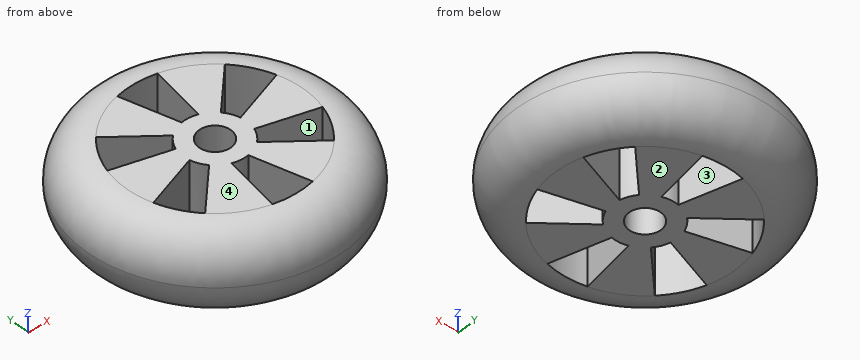
from build123d import *

# Parameters (mm, degrees)
SKETCH_1_R               = 32.5
SKETCH_1_R_2             = 4
EXTRUDE_1_DEPTH          = 20
FILLET_1_R               = 10
CUT_EXTRUDE_1_DEPTH      = 20
PATTERN_CIRCULAR_1_COUNT = 6


with BuildPart() as part:
    # 草图1 → 凸台-拉伸1 (new body)
    with BuildSketch(Plane.XY):
        Circle(SKETCH_1_R)
        Circle(SKETCH_1_R_2, mode=Mode.SUBTRACT)
    extrude(amount=EXTRUDE_1_DEPTH)

    # 圆角1
    fillet_1_edges = [part.edges().sort_by_distance(p)[0] for p in [
        (-32.5, 0, 0),
        (-32.5, 0, 20),
    ]]
    fillet(fillet_1_edges, radius=FILLET_1_R - 0.0001)  # a hair under: the kernel refuses the full size

    # 草图2 → 切除-拉伸1 (cut)
    with BuildSketch(Plane.XY.offset(20)):
        with BuildLine():
            Line((-5.142061575, 21.884386505), (-1.389185421, 7.878462024))
            ThreePointArc((-1.389185421, 7.878462024), (0.633872, 7.974848355), (2.616301677, 7.560090313))
            Line((2.616301677, 7.560090313), (5.142061575, 21.884386505))
            ThreePointArc((5.142061575, 21.884386505), (0, 22.480372994), (-5.142061575, 21.884386505))
        make_face()
    cut_extrude_1 = extrude(amount=-CUT_EXTRUDE_1_DEPTH, mode=Mode.SUBTRACT)

    # 阵列(圆周)1: 切除-拉伸1 ×6 about axis
    pattern_circular_1_axis = Axis((0, 0, 0), (0, 0, 1))
    for i in range(1, PATTERN_CIRCULAR_1_COUNT):
        add(cut_extrude_1.rotate(pattern_circular_1_axis, i * 360 / PATTERN_CIRCULAR_1_COUNT), mode=Mode.SUBTRACT)


solid = part.part
Build history of the part. All positions in model axes, mm. Face numbers are marked on the shaded views. A direction names the side the tool comes from. Round coordinates to 2 decimals unless told otherwise and drop trailing zeros. Loops run counter-clockwise (first coordinate to the right, second up) from the corner with the lowest first, then second, coordinate; pieces in that order, holes last. Notation, with made-up numbers: (22.25, 18.5) -> (65.25, 18.5) arc R25 ccw to (65.25, 38.5) -> close; hole circle Ø5 at (88.25, 13.5). An arc over 180 degrees is marked (long way). Answer in a Markdown table with one row per item.
Item 1: Saw through at B-B (x = 0). State how many separate pieces and enclosed holes the cut face has, and give its area (3 significant figures).
Answers below:
| item | result |
|---|---|
| separate pieces | 4 |
| enclosed holes | 0 |
| area | 475 mm² |
Item 2: Which spindle directions (+Z, -Z, +X, -X, +Y, -Y) get a long thin tool onto all of the face, cutting with end or side? Do the marked faces 3 and 4. Say none if no direction does.
Answers below:
| item | result |
|---|---|
| face 3 | +Z, -Z |
| face 4 | +Z, +X, -X, +Y, -Y |
Item 3: Drill centre lines: L1, parallel to Y at x = 10.5, z = 14; L2, parallel to Y at x = 1, z = 1.25; L3, parallel to Y at x = -15, z = 8.5. Where is each one in solid material? Low to high. Write a range as [from, to].
Answers below:
| item | result |
|---|---|
| L1 | y = [-29.87, -10.46], [-3.54, 2.48], [9.51, 29.87] |
| L2 | y = [-27.32, -22.46], [-7.94, -3.87], [3.87, 7.94], [22.46, 27.32] |
| L3 | y = [-28.7, -14.01], [-4.11, 4.74], [14.24, 28.7] |
Item 4: Pin check, flat tips, straight feed: pin 1 (9 mm diameter, centred on x = 0, y = 0, fed in from +Z); pin 2 (8 mm diameter, centred on y = 4, z = 7.5, fed in from +X); pin 3 (5 mm diameter, centred on x = -22.5, z = 18, fed in from +Y); pin 4 (4 mm diameter, centred on y = -9, z = 3, fed in from +X). Stop position of each tip, or through.
Answers below:
| item | result |
|---|---|
| pin 1 | stops at z = 20 |
| pin 2 | stops at x = 32.49 |
| pin 3 | stops at y = 22.13 |
| pin 4 | stops at x = 29.96 |
Item 5: Saw through at C-C (z = 7.5). Write the cut outline in (x, y), and give its area (3 significant figures).
Answers below:
| item | result |
|---|---|
| outline | circle Ø64.36 at (0, 0); hole (-21.52, -6.49) arc R22.48 ccw to (-16.38, -15.4) -> (-6.13, -5.14) arc R8 cw to (-7.86, -1.51) -> close; hole (-21.52, 6.49) -> (-7.52, 2.74) arc R8 cw to (-5.24, 6.05) -> (-16.38, 15.4) arc R22.48 ccw to start; hole (-5.14, -21.88) arc R22.48 ccw to (5.14, -21.88) -> (1.39, -7.88) arc R8 cw to (-2.62, -7.56) -> close; hole (-5.14, 21.88) -> (-1.39, 7.88) arc R8 cw to (2.62, 7.56) -> (5.14, 21.88) arc R22.48 ccw to start; hole circle Ø8 at (0, 0); hole (5.24, -6.05) -> (16.38, -15.4) arc R22.48 ccw to (21.52, -6.49) -> (7.52, -2.74) arc R8 cw to start; hole (6.13, 5.14) arc R8 cw to (7.86, 1.51) -> (21.52, 6.49) arc R22.48 ccw to (16.38, 15.4) -> close |
| area | 2,580 mm² |
Item 6: Mould opens along X. For the marked faces 1 and 2 say: +X half, -X half, draft (parallel to the pull), parting line (faces both ways), or undercut.
Answers below:
| item | result |
|---|---|
| face 1 | undercut |
| face 2 | draft |
